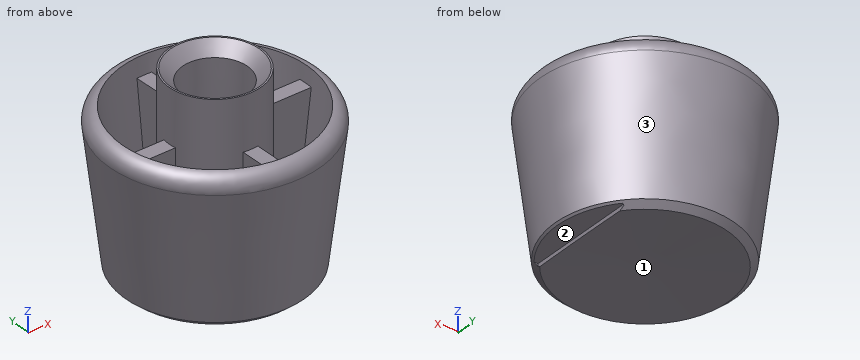
from build123d import *

# Parameters (mm, degrees)
F3_DEPTH  = 3.175
F5_DEPTH  = 3.175
F7_DEPTH  = 3.175
F8_SIZE   = 2.54
F9_SIZE   = 5.08
F10_W     = 12.513392
F10_H     = 47.661307
F11_DEPTH = 25.4


with BuildPart() as f1:
    # F0 (on Front) → F1 (revolve)
    with BuildSketch(Plane.XZ):
        with BuildLine():
            Line((0, 19.05), (0, 0))
            Line((0, 0), (0, -0.913425))
            Line((0, -0.913425), (38.565893, -1.763764))
            Line((38.565893, -1.763764), (45.640576, 56.988166))
            ThreePointArc((45.640576, 56.988166), (44.387599, 61.595058), (40.279133, 64.026912))
            Line((40.279133, 64.026912), (34.23503, 13.833469))
            ThreePointArc((34.23503, 13.833469), (31.941065, 9.669371), (27.399097, 8.264908))
            Line((27.399097, 8.264908), (25.775305, 8.401293))
            ThreePointArc((25.775305, 8.401293), (21.632523, 10.430895), (19.956781, 14.729012))
            Line((19.956781, 14.729012), (19.956781, 28.661031))
            Line((19.956781, 28.661031), (19.956781, 79.461031))
            Line((19.956781, 79.461031), (14.187589, 79.461031))
            Line((14.187589, 79.461031), (13.97, 19.05))
            Line((13.97, 19.05), (0, 19.05))
        make_face()
    revolve(axis=Axis((0, 0, 9.525), (0, 0, 1)))

    # F2 (on Front) → F3 (join, symmetric)
    with BuildSketch(Plane.XZ):
        Polygon((-17.64158, 56.308575), (-40.932791, 56.308575), (-36.213137, 2.431753), (-36.199561, 2.276776), (-17.64158, 1.878101), align=None)
    extrude(amount=F3_DEPTH, both=True)

    # F4 (on Front) → F5 (join, symmetric)
    with BuildSketch(Plane.XZ):
        Polygon((42.761714, 57.315655), (16.789319, 57.315655), (16.789319, 0.20661), (35.935931, 0.20661), align=None)
    extrude(amount=F5_DEPTH, both=True)

    # F6 (on Right) → F7 (join, symmetric)
    with BuildSketch(Plane.YZ):
        Polygon((-16.432097, 1.235654), (-16.432097, 56.315523), (-41.003351, 56.652121), (-34.406153, 1.235654), align=None)
        Polygon((42.709365, 56.236618), (17.860977, 56.908193), (17.860977, 0.033839), (35.461162, -0.207263), align=None)
    extrude(amount=F7_DEPTH, both=True)

    # F8
    f8_edges = [f1.edges().sort_by_distance(p)[0] for p in [
        (-38.565893, 0, -1.763764),
    ]]
    chamfer(f8_edges, length=F8_SIZE)

    # F9
    f9_edges = [f1.edges().sort_by_distance(p)[0] for p in [
        (-14.187589, 0, 79.461031),
        (-13.97, 0, 19.05),
        (14.078795, 0, 49.255515),
    ]]
    chamfer(f9_edges, length=F9_SIZE)

    # F10 (on Top) → F11 (cut)
    with BuildSketch(Plane.XY):
        with Locations((34.57921, 0.681657)):
            Rectangle(F10_W, F10_H)
    extrude(amount=-F11_DEPTH, mode=Mode.SUBTRACT)


solid = f1.part
Verification items for the finished model (mm, model axes). Face numbers are marked on the shaded views. Coordinates: 2 decimals unless noted, no trailing zeros. Order: outer loops, then holes, each group sorted by start corner. A loop starts at its lowest first (then second) coordinate and runs counter-clockwise, first axis right, second up. Notation, with made-up numbers: (-22, 49) -> (-9, 49) arc R21 ccw to (-9, 65) -> close; hole circle Ø9 at (13.5, 79.5). An arc over 180 degrees is marked (long way). Use CSV: the item, a comma, the result in double quotes. Start each with the question number.
Q1. Section check B-B, the plane z = 27.5. Record the cut outline in (x, y) (3 decimals).
Q2. Depth check by flat-ended pin: P1, Ø5, axis at x = 7, z = 68.5, coming from the -Y side; P2, Ø5.5, axis at x = -3.5, y = 0.5, coming from the +Z side; P3, Ø1.9, axis at y = 9.5, z = -0.5, coming from the +X side. Enter the tip coordinate at first touch or a pass-through.
Q3. Section check C-C, the plane z = 46. Record the cut outline in (x, y) (3 decimals).
Q4. Section check A-A, the plane z = 11.5. Record the cut outline in (x, y) (3 decimals).
Q5. Draft check along X on the marked faces 1, 2 and 3. Enter one of: +X half, -X half, draft (parallel to the pull), parting line (faces both ways), or undercut.
Q6. Thickness scan on line 1 along Y through (x, z) = (-9, 41); line 2 along X through (y, z) = (-20, 52) (3 decimals); line 3 along X through (y, z) = (10.5, 22.5). Record the ranges inside material, lowest first.
Returned:
1,outline,"circle Ø84.179 at (0, 0); hole (-35.74, -3.175) arc R35.881 ccw to (-3.175, -35.74) -> (-3.175, -19.703) arc R19.957 cw to (-19.703, -3.175) -> close; hole (-35.74, 3.175) -> (-19.703, 3.175) arc R19.957 cw to (-3.175, 19.703) -> (-3.175, 35.74) arc R35.881 ccw to start; hole circle Ø28.001 at (0, 0); hole (3.175, -35.74) arc R35.881 ccw to (35.74, -3.175) -> (19.703, -3.175) arc R19.957 cw to (3.175, -19.703) -> close; hole (3.175, 19.703) arc R19.957 cw to (19.703, 3.175) -> (35.74, 3.175) arc R35.881 ccw to (3.175, 35.74) -> close"
2,P1,"stops at y = -19.44"
2,P2,"stops at z = 19.05"
2,P3,"stops at x = 37.35"
3,outline,"circle Ø88.635 at (0, 0); hole (-37.976, -3.175) arc R38.108 ccw to (-3.175, -37.976) -> (-3.175, -19.703) arc R19.957 cw to (-19.703, -3.175) -> close; hole (-37.976, 3.175) -> (-19.703, 3.175) arc R19.957 cw to (-3.175, 19.703) -> (-3.175, 37.976) arc R38.108 ccw to start; hole circle Ø28.134 at (0, 0); hole (3.175, -37.976) arc R38.108 ccw to (37.976, -3.175) -> (19.703, -3.175) arc R19.957 cw to (3.175, -19.703) -> close; hole (3.175, 19.703) arc R19.957 cw to (19.703, 3.175) -> (37.976, 3.175) arc R38.108 ccw to (3.175, 37.976) -> close"
4,outline,"circle Ø80.326 at (0, 0); hole (-33.326, -3.175) arc R33.477 ccw to (-3.175, -33.326) -> (-3.175, -20.596) arc R20.839 cw to (-20.596, -3.175) -> close; hole (-33.326, 3.175) -> (-20.596, 3.175) arc R20.839 cw to (-3.175, 20.596) -> (-3.175, 33.326) arc R33.477 ccw to start; hole (3.175, -33.326) arc R33.477 ccw to (33.326, -3.175) -> (20.596, -3.175) arc R20.839 cw to (3.175, -20.596) -> close; hole (3.175, 20.596) arc R20.839 cw to (20.596, 3.175) -> (33.326, 3.175) arc R33.477 ccw to (3.175, 33.326) -> close"
5,face 1,"undercut"
5,face 2,"draft"
5,face 3,"parting line"
6,line 1,"y = -42.78 to -36.41, -17.81 to -10.79, 10.79 to 17.81, 36.41 to 42.78"
6,line 2,"x = -40.356 to -33.284, -3.175 to 3.175, 33.284 to 40.356"
6,line 3,"x = -40.14 to -33.68, -16.97 to -6.51, 6.51 to 16.97, 33.68 to 40.14"
